For this review, take the finished solid that the model builds, in its own axes (mm). Round coordinates to 2 decimals unless told otherwise and drop trailing zeros. Write each loop counter-clockwise with the first axis right and the second up, starting at its lowest first coordinate (ties: lowest second). Pieces come first, ordered by that corner, then holes. Notation, with made-up numbers: (-13.5, -31.75) -> (37.5, -31.75) arc R28 ccw to (37.5, 0.25) -> close; hole circle Ø1 at (4, -38). An arc over 180 degrees is marked (long way). Answer in a Markdown table with one row per item.
from build123d import *

# Parameters (mm, degrees)
BOSS_EXTRUDE1_DEPTH = 1.25
CUT_EXTRUDE1_DEPTH  = 0.6


with BuildPart() as part:
    # Sketch1 → Boss-Extrude1 (new body)
    with BuildSketch(Plane(origin=(0, 0, 0), x_dir=(1, 0, 0), z_dir=(0, 1, 0))):
        Polygon((0, 58), (0, 124.3), (2, 124.3), (2, 127.3), (0, 127.3), (0, 137.3), (41, 137.3), (41, 127.3), (39, 127.3), (39, 124.3), (41, 124.3), (41, 58), (39, 58), (39, 55), (41, 55), (41, 5), (39, 5), (39, 0), (26.5, 0), (26.5, 12), (14.5, 12), (14.5, 0), (2, 0), (2, 5), (0, 5), (0, 55), (2, 55), (2, 58), align=None)
    extrude(amount=BOSS_EXTRUDE1_DEPTH)

    # Sketch2 → Cut-Extrude1 (cut)
    with BuildSketch(Plane(origin=(0, 1.25, 0), x_dir=(1, 0, 0), z_dir=(0, 1, 0))):
        Polygon((5, 132.3), (36, 132.3), (36, 17), (36, 5), (29.5, 5), (29.5, 17), (11.5, 17), (11.5, 5), (5, 5), (5, 17), align=None)
    extrude(amount=-CUT_EXTRUDE1_DEPTH, mode=Mode.SUBTRACT)


solid = part.part
1) Consider section B-B on y = 0.35. State the section outline as (x, z) points.
Solved:
| item | result |
|---|---|
| outline | (0, -137.3) -> (41, -137.3) -> (41, -127.3) -> (39, -127.3) -> (39, -124.3) -> (41, -124.3) -> (41, -58) -> (39, -58) -> (39, -55) -> (41, -55) -> (41, -5) -> (39, -5) -> (39, 0) -> (26.5, 0) -> (26.5, -12) -> (14.5, -12) -> (14.5, 0) -> (2, 0) -> (2, -5) -> (0, -5) -> (0, -55) -> (2, -55) -> (2, -58) -> (0, -58) -> (0, -124.3) -> (2, -124.3) -> (2, -127.3) -> (0, -127.3) -> close |
2) Consider section C-C on z = -98.5. State the section outline as (x, y) points, then the cut area to 4 significant figures.
Solved:
| item | result |
|---|---|
| outline | (0, 0) -> (41, 0) -> (41, 1.25) -> (36, 1.25) -> (36, 0.65) -> (5, 0.65) -> (5, 1.25) -> (0, 1.25) -> close |
| area | 32.65 mm² |
3) Consider section A-A on x = 32.5. State the section outline as (y, z) points.
Solved:
| item | result |
|---|---|
| outline | (0, -137.3) -> (1.25, -137.3) -> (1.25, -132.3) -> (0.65, -132.3) -> (0.65, -5) -> (1.25, -5) -> (1.25, 0) -> (0, 0) -> close |
4) For line 1 (Z direction, x = 39.5, y = 0.85); line 2 (X direction, y = 0.9, z = -47.5); line 3 (Z direction, x = 17, y = 0.75), list the stretches that pass through material, from the lowest coordinate up. Write a range as [from, to].
Solved:
| item | result |
|---|---|
| line 1 | [-137.3, -127.3], [-124.3, -58], [-55, -5] |
| line 2 | [0, 5], [36, 41] |
| line 3 | [-137.3, -132.3], [-17, -12] |
5) Mouldability with a two-part tool opening along X and no side actions: class faces 1 (the flat face through (21, 0.65, -70)), 2 (the flat face through (21, 0, -70)) as pulls with the +X half, pulls with the -X half, needs draft (parallel to the pull), parting line crosses it, or undercut.
Solved:
| item | result |
|---|---|
| face 1 | undercut |
| face 2 | needs draft |
6) Clearance check with flat-ended pins moving along their axes: pin 1 Ø0.6 at (y, z) = (1, -2) entering from -X; pin 2 Ø10 at (x, z) = (27, -66) entering from +Y. State where each tip first meets the part, or that it passes through.
Solved:
| item | result |
|---|---|
| pin 1 | x = 2 |
| pin 2 | y = 0.65 |
